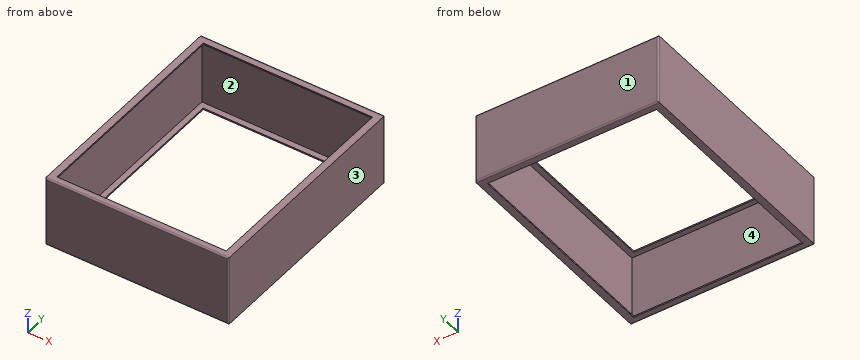
```python
from build123d import *

# Parameters (mm, degrees)
SKETCH2_W           = 330.2
SKETCH2_H           = 406.4
BOSS_EXTRUDE1_DEPTH = 127
FILLET1_R           = 2.54
FILLET2_R           = 2.54
SKETCH3_W           = 304.8
SKETCH3_H           = 381
CUT_EXTRUDE1_DEPTH  = 127
SHELL4_START        = 2.54
SHELL4_OUTLINE_W    = 401.32
SHELL4_OUTLINE_H    = 121.92
SHELL4_DEPTH        = 325.12


# Read off the part's stored shape, not the designer's step: Shell4
with BuildPart() as part:
    # Sketch2 → Boss-Extrude1 (new body)
    with BuildSketch(Plane.XY):
        with Locations((165.1, 203.2)):
            Rectangle(SKETCH2_W, SKETCH2_H)
    extrude(amount=BOSS_EXTRUDE1_DEPTH)

    # Fillet1
    fillet1_edges = [part.edges().sort_by_distance(p)[0] for p in [
        (165.1, 406.4, 127),
        (165.1, 406.4, 0),
        (0, 406.4, 63.5),
        (330.2, 406.4, 63.5),
    ]]
    fillet(fillet1_edges, radius=FILLET1_R)

    # Fillet2
    fillet2_edges = [part.edges().sort_by_distance(p)[0] for p in [
        (165.1, 0, 0),
        (330.2, 0, 63.5),
        (0, 0, 63.5),
        (165.1, 0, 127),
    ]]
    fillet(fillet2_edges, radius=FILLET2_R)

    # Sketch3 → Cut-Extrude1 (cut)
    with BuildSketch(Plane.XY.offset(127)):
        with Locations((165.1, 202.565)):
            Rectangle(SKETCH3_W, SKETCH3_H)
    extrude(amount=-CUT_EXTRUDE1_DEPTH, mode=Mode.SUBTRACT)

    # Shell4 outline → Shell4 (cut)
    with BuildSketch(Plane.YZ.offset(SHELL4_START)):
        with Locations((203.2, 63.5)):
            Rectangle(SHELL4_OUTLINE_W, SHELL4_OUTLINE_H)
    extrude(amount=SHELL4_DEPTH, mode=Mode.SUBTRACT)


solid = part.part
```
Work out the finished part from the listing and answer in its coordinate system (mm). Face numbers are marked on the shaded views. A direction names the side the tool comes from. Round coordinates to 2 decimals unless told otherwise and drop trailing zeros. Loops run counter-clockwise (first coordinate to the right, second up) from the corner with the lowest first, then second, coordinate; pieces in that order, holes last. Notation, with made-up numbers: M 17.5,34 L 75.5,34 A24 ccw 75.5,69 Z; hole C 24,-39 d4. An arc over 180 degrees is marked long. One line per question, with ' | ' between items.
Q1. Find section B-B, the plane y = 85. Give the vertices of the cut face in (x, z), then the cut area to 3 significant figures.
Conclusion:
outline: M 0,0 L 12.7,0 L 12.7,2.54 L 2.54,2.54 L 2.54,124.46 L 12.7,124.46 L 12.7,127 L 0,127 Z; M 317.5,0 L 330.2,0 L 330.2,127 L 317.5,127 L 317.5,124.46 L 327.66,124.46 L 327.66,2.54 L 317.5,2.54 Z | area: 748 mm2
Q2. A tool of negligible diameter and unlimited length cuts with its end or side. For the marked faces 1 and 2, from which of +Z, -Z, +X, -X, +Y, -Y can it reach the whole face along a straight path? Write none if from no direction.
Conclusion:
face 1: +Z, -Z, +X, -X, +Y | face 2: none
Q3. Find section C-C, the plane z = 89. Give the vertices of the cut face in (x, y), then the cut area to 3 significant figures.
Conclusion:
outline: M 0,2.54 A2.54 ccw 2.54,0 L 327.66,0 A2.54 ccw 330.2,2.54 L 330.2,403.86 A2.54 ccw 327.66,406.4 L 2.54,406.4 A2.54 ccw 0,403.86 Z; hole M 2.54,2.54 L 327.66,2.54 L 327.66,403.86 L 2.54,403.86 Z | area: 3,710 mm2
Q4. The mould has two halves that part along Z. Classify the marked faces 3 and 4: +Z half, -Z half, draft (parallel to the pull), parting line (faces both ways), or undercut.
Conclusion:
face 3: draft | face 4: undercut
Q5. Consider line 1 along X through (y, z) = (84.5, 56); line 2 along Y through (x, z) = (174.5, 73). Determine where each line is inside the solid, lowest interval first. Write a range as from..to.
Conclusion:
line 1: x = 0..2.54, 327.66..330.2 | line 2: y = 0..2.54, 403.86..406.4
Q6. Find section A-A, the plane x = 301.5. Give the vertices of the cut face in (y, z) (3 decimals), then the cut area to 3 significant figures.
Conclusion:
outline: M 0,2.54 A2.54 ccw 2.54,0 L 12.065,0 L 12.065,2.54 L 2.54,2.54 L 2.54,124.46 L 12.065,124.46 L 12.065,127 L 2.54,127 A2.54 ccw 0,124.46 Z; M 393.065,0 L 403.86,0 A2.54 ccw 406.4,2.54 L 406.4,124.46 A2.54 ccw 403.86,127 L 393.065,127 L 393.065,124.46 L 403.86,124.46 L 403.86,2.54 L 393.065,2.54 Z | area: 743 mm2
Q7. Each of these flat-tipped pins is pushed along its axis until it touches: pin 1 Ø0.8 at (x, z) = (173, 125.5) entering from -Y; pin 2 Ø1.3 at (x, z) = (108, 126) entering from +Y; pin 3 Ø3 at (x, z) = (124.5, 1.5) entering from -Y; pin 4 Ø1.3 at (x, z) = (189, 1.5) entering from +Y. Where does it stop, or does it pass through?
Conclusion:
pin 1: stops at y = 0.08 | pin 2: stops at y = 406.24 | pin 3: stops at y = 0 | pin 4: stops at y = 406.37
